from build123d import *

# Parameters (mm, degrees)
BOSS_EXTRUDE1_DEPTH  = 3.175
M5_CLEARANCE_HOLE1_D = 5.5
LPATTERN1_COUNT      = 3
LPATTERN1_PITCH      = 20
LPATTERN2_COUNT      = 3
LPATTERN2_PITCH      = 20


with BuildPart() as part:
    # Sketch1 → Boss-Extrude1 (new body)
    with BuildSketch(Plane.XY):
        Polygon((0, 0), (0, 60), (20, 60), (60, 20), (60, 0), align=None)
    extrude(amount=BOSS_EXTRUDE1_DEPTH)

    # M5 Clearance Hole1 (through all)
    with Locations(Plane(origin=(10, 10, 3.175), x_dir=(1, 0, 0), z_dir=(0, 0, 1))):
        with Locations((0, 0)):
            m5_clearance_hole1 = Hole(M5_CLEARANCE_HOLE1_D / 2)

    # LPattern1: M5 Clearance Hole1 ×3
    with Locations(*[(i * LPATTERN1_PITCH, 0, 0) for i in range(1, LPATTERN1_COUNT)]):
        add(m5_clearance_hole1, mode=Mode.SUBTRACT)

    # LPattern2: M5 Clearance Hole1 ×3
    with Locations(*[(0, i * LPATTERN2_PITCH, 0) for i in range(1, LPATTERN2_COUNT)]):
        add(m5_clearance_hole1, mode=Mode.SUBTRACT)


solid = part.part
The model under review builds one solid part; all positions refer to its coordinate system, in mm. Round coordinates to 2 decimals unless told otherwise and drop trailing zeros. Write each loop counter-clockwise with the first axis right and the second up, starting at its lowest first coordinate (ties: lowest second). Pieces come first, ordered by that corner, then holes. Notation, with made-up numbers: M 19,54 L 45,54 A15 ccw 45,66 Z; hole C 62,21.5 d9. An arc over 180 degrees is marked long. Use a Markdown table: item, result. Add a question column.
Q1. We need section D-D, the plane x = 10. State the section outline as (y, z) points (3 decimals).
Q2. We need section A-A, the plane y = 30. State the section outline as (x, z) points (3 decimals).
Q3. Insertion check: pin 1 (5 mm diameter, centred on x = 30, y = 10, fed in from -Z). The pin has a flat end and moves straight along its axis. Give the tip position at first contact, or say it passes through.
Q4. To check wall thickness, follow line 1 (Y direction, x = 10, z = 2.15); line 2 (Y direction, x = 30, z = 1.6); line 3 (Y direction, x = 31.5, z = 1.15). State the ranges of each line that lie inside material, in increasing order.
Q5. We need section B-B, the plane x = 50. State the section outline as (y, z) points (3 decimals).
Q6. The part is to be moulded in two halves that separate along X. For faces 1 (the face through (10.358, 52.727, 1.565)), 2 (the face through (8.52, 12.32, 1.57)), 3 (the face through (10, 60, 2)), 4 (the face through (40, 40, 2)), say which applies: pulls with the +X half, pulls with the -X half, needs draft (parallel to the pull), parting line crosses it, or undercut.
Q7. We need section C-C, the plane z = 0.8. State the section outline as (x, y) points, plus the area to 3 significant figures.
Findings below:
| question | item | result |
|---|---|---|
| 1 | outline | M 0,0 L 7.25,0 L 7.25,3.175 L 0,3.175 Z; M 12.75,0 L 27.25,0 L 27.25,3.175 L 12.75,3.175 Z; M 32.75,0 L 47.25,0 L 47.25,3.175 L 32.75,3.175 Z; M 52.75,0 L 60,0 L 60,3.175 L 52.75,3.175 Z |
| 2 | outline | M 0,0 L 7.25,0 L 7.25,3.175 L 0,3.175 Z; M 12.75,0 L 50,0 L 50,3.175 L 12.75,3.175 Z |
| 3 | pin 1 | passes through |
| 4 | line 1 | y = 0 to 7.25, 12.75 to 27.25, 32.75 to 47.25, 52.75 to 60 |
| 4 | line 2 | y = 0 to 7.25, 12.75 to 50 |
| 4 | line 3 | y = 0 to 7.7, 12.3 to 48.5 |
| 5 | outline | M 0,0 L 7.25,0 L 7.25,3.175 L 0,3.175 Z; M 12.75,0 L 30,0 L 30,3.175 L 12.75,3.175 Z |
| 6 | face 1 | undercut |
| 6 | face 2 | undercut |
| 6 | face 3 | needs draft |
| 6 | face 4 | pulls with the +X half |
| 7 | outline | M 0,0 L 60,0 L 60,20 L 20,60 L 0,60 Z; hole C 10,10 d5.5; hole C 10,30 d5.5; hole C 10,50 d5.5; hole C 30,10 d5.5; hole C 50,10 d5.5 |
| 7 | area | 2,680 mm² |
